Verification items for the finished model (mm, model axes). A direction names the side the tool comes from. Round coordinates to 2 decimals unless told otherwise and drop trailing zeros. Write each loop counter-clockwise with the first axis right and the second up, starting at its lowest first coordinate (ties: lowest second). Pieces come first, ordered by that corner, then holes. Notation, with made-up numbers: (51, -1.5) - (71, -1.5) arc R11 ccw to (71, 16.5) - close; hole circle Ø10 at (72, 44). An arc over 180 degrees is marked (long way). Answer as a JSON object with one key per item and string values.
```python
from build123d import *

# Parameters (mm, degrees)
F0_W         = 14
F0_H         = 17.5
F1_DEPTH     = 3.7
F3_DEPTH     = 5.4
F4_R         = 3.69999
F5_R         = 3
F6_T1_DEPTH  = 7.30001
F6_T3_DEPTH  = 5.00001
F6_T5_DEPTH  = 19.5
F6_T8_ANGLE  = 90
F6_T10_ANGLE = 90


# Not quite as in the source:
# - a fillet or chamfer that OpenCascade refuses, or shapes differently, is made with other operations: its cross-section is extruded or revolved along the edge and cut away or added
# - a fillet or chamfer is up to 0.001 mm smaller than in the source, because OpenCascade refuses the exact size


with BuildPart() as f1:
    # F0 (on Top) → F1 (new body)
    with BuildSketch(Plane.XY):
        with Locations((-0.4103374667, 3.4223956802)):
            Rectangle(F0_W, F0_H)
    extrude(amount=F1_DEPTH)

    # F2 (on face) → F3 (cut)
    with BuildSketch(Plane.XY.offset(3.7)):
        with BuildLine():
            Line((-5.3451164257, 9.1307080224), (-5.3451164257, 9.2324278445))
            ThreePointArc((-5.3451164257, 9.2324278445), (-5.3456139214, 9.1815679334), (-5.3451164257, 9.1307080224))
        make_face()
        with BuildLine():
            Line((-5.3451164257, 12.1723956802), (-5.3451164257, 9.2324278445))
            Line((-5.3451164257, 9.2324278445), (-5.3451164257, 9.1307080224))
            ThreePointArc((-5.3451164257, 9.1307080224), (-2.7588797704, 6.5816017765), (-0.1467657558, 9.1041843944))
            Line((-0.1467657558, 9.1041843944), (-0.055406418, 12.1723956802))
            Line((-0.055406418, 12.1723956802), (-5.3451164257, 12.1723956802))
        make_face()
    extrude(amount=-F3_DEPTH, mode=Mode.SUBTRACT)

    # F4 (radius 3.7 in the source; OpenCascade refuses exactly that, so slightly less here)
    f4_edges = [f1.edges().sort_by_distance(p)[0] for p in [
        (6.589663, 3.422396, 0),
    ]]
    fillet(f4_edges, radius=F4_R)

    # F5
    f5_edges = [f1.edges().sort_by_distance(p)[0] for p in [
        (-7.410337, -5.327604, 1.85),
    ]]
    fillet(f5_edges, radius=F5_R)

    # F6: fillet of radius 2 on 1 edges, made by hand

    # F6_s2 → F6_t1 (cut)
    with BuildSketch(Plane.YZ.offset(-4.4103374667)):
        with BuildLine():
            ThreePointArc((-5.3276043198, 2), (-4.7418178821, 0.5857864376), (-3.3276043198, 0))
            Line((-3.3276043198, 0), (-5.3276043198, 0))
            Line((-5.3276043198, 0), (-5.3276043198, 2))
        make_face()
    extrude(amount=F6_T1_DEPTH, mode=Mode.SUBTRACT)

    # F6_s4 → F6_t3 (cut)
    with BuildSketch(Plane.XY.offset(3.69999)):
        with BuildLine():
            ThreePointArc((4.5896625333, -5.3276043198), (6.0038760956, -4.7418178821), (6.5896625333, -3.3276043198))
            Line((6.5896625333, -3.3276043198), (6.5896625333, -5.3276043198))
            Line((6.5896625333, -5.3276043198), (4.5896625333, -5.3276043198))
        make_face()
    extrude(amount=F6_T3_DEPTH, mode=Mode.SUBTRACT)

    # F6_s6 → F6_t5 (cut)
    with BuildSketch(Plane.XZ.offset(-17.1723956802)):
        with BuildLine():
            ThreePointArc((-5.4103374667, 0), (-6.8245510291, 0.5857864376), (-7.4103374667, 2))
            Line((-7.4103374667, 2), (-7.4103374667, 0))
            Line((-7.4103374667, 0), (-5.4103374667, 0))
        make_face()
    extrude(amount=F6_T5_DEPTH, mode=Mode.SUBTRACT)

    # F6_s7 → F6_t8 (revolve, cut)
    with BuildSketch(Plane.YZ.offset(2.8896725333)):
        with BuildLine():
            ThreePointArc((-5.3276043198, 2), (-4.7418178821, 0.5857864376), (-3.3276043198, 0))
            Line((-3.3276043198, 0), (-5.3276043198, 0))
            Line((-5.3276043198, 0), (-5.3276043198, 2))
        make_face()
    revolve(axis=Axis((2.8896725333, -5.3276043198, 3.69999), (0, -1, 0)), revolution_arc=F6_T8_ANGLE, mode=Mode.SUBTRACT)

    # F6_s9 → F6_t10 (revolve, cut)
    with BuildSketch(Plane.YZ.offset(-4.4103374667)):
        with BuildLine():
            ThreePointArc((-5.3276043198, 2), (-4.7418178821, 0.5857864376), (-3.3276043198, 0))
            Line((-3.3276043198, 0), (-5.3276043198, 0))
            Line((-5.3276043198, 0), (-5.3276043198, 2))
        make_face()
    revolve(axis=Axis((-4.4103374667, -2.3276043198, 0), (0, 0, -1)), revolution_arc=F6_T10_ANGLE, mode=Mode.SUBTRACT)


solid = f1.part
```
1. Access from +Z, -Z, +X, -X, +Y, -Y to the whole of each face (thin tool, end or side, straight path). Record for faces 1 (the face through (-0.811, -4.757, 0.601)), 2 (the face through (-5.345, 11, 2)).
Completed:
{"face 1": "-Z, +X, -X, -Y", "face 2": "+Z, -Z, +Y"}
2. Cross-section at C-C (x = -3.5). Record the boundary of the cut face in (y, z).
Completed:
{"outline": "(-5.33, 2) arc R2 ccw to (-3.33, 0) - (6.69, 0) - (6.69, 3.7) - (-5.33, 3.7) - close"}
3. Cross-section at D-D (x = -1.25). Record the boundary of the cut face in (y, z), plus the area to 3 significant figures.
Completed:
{"outline": "(-5.33, 2) arc R2 ccw to (-3.33, 0) - (7.05, 0) - (7.05, 3.7) - (-5.33, 3.7) - close", "area": "45.0 mm^2"}
4. Material ranges on probe 1 along Z at (x, y) = (3, -3); probe 2 along X at (y, z) = (9.75, 3.1); probe 3 along X at (y, z) = (-2.25, 0.9), recorded low to high. Write a range as from..to.
Completed:
{"probe 1": "z = 0..3.7", "probe 2": "x = -7.41..-5.35, -0.13..6.54", "probe 3": "x = -7.08..5.31"}
5. Go/stop test with flat-tipped pins: pin 1 (1.5 mm diameter, centred on y = 11, z = 2.5, fed in from +X); pin 2 (1.5 mm diameter, centred on y = 6.5, z = 1, fed in from -X). Record where each tip stops, or that it passes through.
Completed:
{"pin 1": "stops at x = 6.56", "pin 2": "stops at x = -7.39"}
